Design review of the part shown in the three views and the two pictorial views. Dimensions are in mm from the part's minimum x, y and z. Give positions to 0.01 mm unless a question says otherwise; leave off trailing zeros. Order: outer loops, then holes, each group sorted by start corner. A loop starts at its lowest first (then second) coordinate and runs counter-clockwise, first axis right, second up. Notation, with made-up numbers: M 30,-18 L 87,-18 A33 ccw 87,14 Z; hole C 88.5,-4 d11. An arc over 180 degrees is marked long. Answer as a JSON object with one key per item and string values.
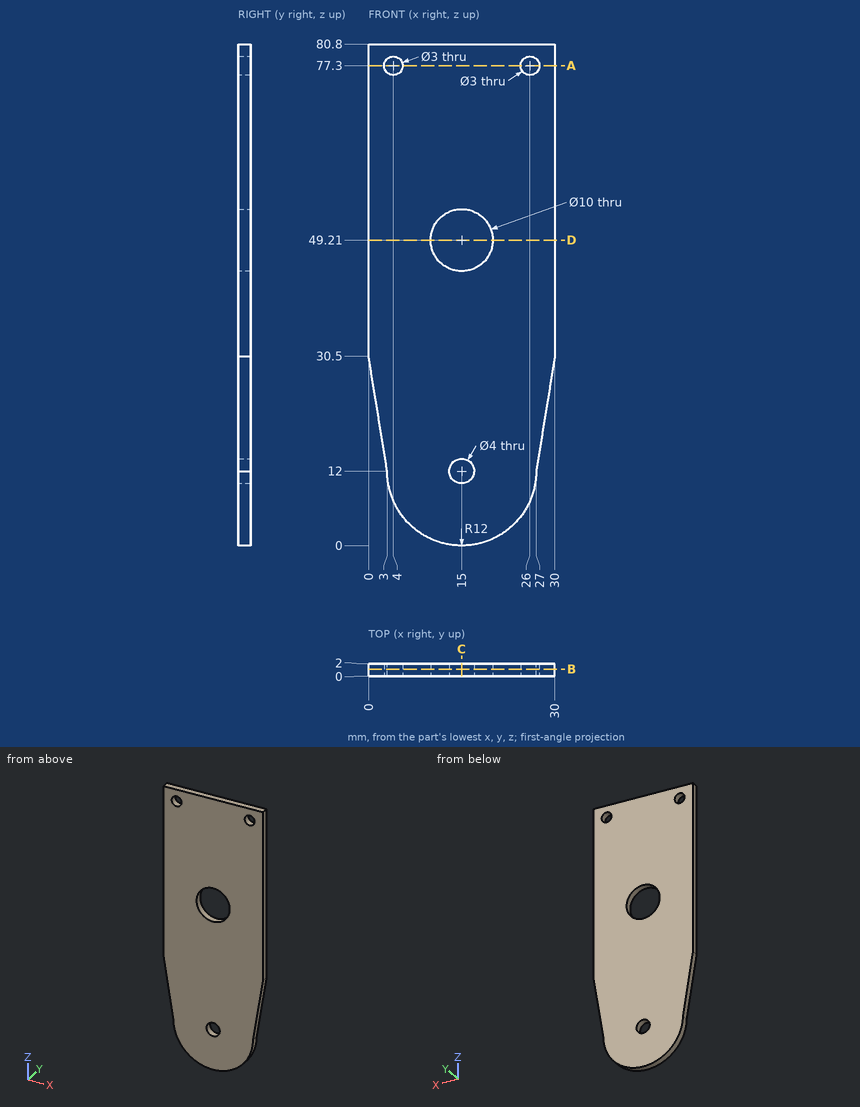
(1) We need section A-A (z = 77.3). Write out the cut boundary in (x, y).
Checked values:
{"outline": "M 0,0 L 2.5,0 L 2.5,2 L 0,2 Z; M 5.5,0 L 24.5,0 L 24.5,2 L 5.5,2 Z; M 27.5,0 L 30,0 L 30,2 L 27.5,2 Z"}
(2) We need section D-D (z = 49.21). Write out the cut boundary in (x, y), plus the area to 3 significant figures.
Checked values:
{"outline": "M 0,0 L 10,0 L 10,2 L 0,2 Z; M 20,0 L 30,0 L 30,2 L 20,2 Z", "area": "40.0 mm^2"}
(3) We need section B-B (y = 1.1). Write out the cut boundary in (x, z), plus the area to 3 significant figures.
Checked values:
{"outline": "M 0,30.5 L 3,12 A12 ccw 27,12 L 30,30.5 L 30,80.8 L 0,80.8 Z; hole C 4,77.3 d3; hole C 15,49.21 d10; hole C 15,12 d4; hole C 26,77.3 d3", "area": "2,130 mm^2"}
(4) To check wall thickness, follow L1, parallel to X at y = 1, z = 77.3; L2, parallel to Z at x = 16.5, y = 1.2; L3, parallel to Z at x = 14, y = 1.75. State the ranges of each line that lie inside material, in increasing order. Write a range as from..to.
Checked values:
{"L1": "x = 0..2.5, 5.5..24.5, 27.5..30", "L2": "z = 0.09..10.68, 13.32..44.44, 53.98..80.8", "L3": "z = 0.04..10.27, 13.73..44.31, 54.11..80.8"}
(5) We need section C-C (x = 15). Write out the cut boundary in (y, z), plus the area to 3 significant figures.
Checked values:
{"outline": "M 0,0 L 2,0 L 2,10 L 0,10 Z; M 0,14 L 2,14 L 2,44.21 L 0,44.21 Z; M 0,54.21 L 2,54.21 L 2,80.8 L 0,80.8 Z", "area": "134 mm^2"}
(6) Insertion check: pin 1 (1 mm diameter, centred on x = 19, y = 0.5, fed in from -Z). The pin has a flat end and moves straight along its axis. Give the tip position at first contact, or say it passes through.
Checked values:
{"pin 1": "stops at z = 0.52"}
